```python
from build123d import *

# Parameters (mm, degrees)
SKETCH1_R                = 1.5
BOSS_EXTRUDE1_DEPTH      = 5
BOSS_EXTRUDE3_START      = -5
SKETCH3_R                = 1.5
BOSS_EXTRUDE3_DEPTH      = 5
BOSS_EXTRUDE5_DEPTH      = 6
BOSS_EXTRUDE5_DEPTH_BACK = 5
BOSS_EXTRUDE5_START      = -3
SKETCH5_R                = 1.5
SKETCH6_W                = 10
SKETCH6_H                = 5.12
CUT_EXTRUDE1_DEPTH       = 10
FILLET1_R                = 5


with BuildPart() as part:
    # Sketch1 → Boss-Extrude1 (new body)
    with BuildSketch(Plane.XY):
        with BuildLine():
            Line((-35.37698341, 4), (-15.37698341, 4))
            ThreePointArc((-15.37698341, 4), (-11.37698341, 0), (-15.37698341, -4))
            Line((-15.37698341, -4), (-35.37698341, -4))
            ThreePointArc((-35.37698341, -4), (-39.37698341, 0), (-35.37698341, 4))
        make_face()
        with Locations((-35.37698341, 0)):
            Circle(SKETCH1_R, mode=Mode.SUBTRACT)
        with Locations((-15.37698341, 0)):
            Circle(SKETCH1_R, mode=Mode.SUBTRACT)
    extrude(amount=BOSS_EXTRUDE1_DEPTH)

    # Sketch3 → Boss-Extrude3 (add)
    with BuildSketch(Plane.XY.offset(5).offset(BOSS_EXTRUDE3_START)):
        with BuildLine():
            Line((-55.37698341, -4), (-35.37698341, -4))
            ThreePointArc((-35.37698341, -4), (-39.37698341, 0), (-35.37698341, 4))
            Line((-35.37698341, 4), (-55.37698341, 4))
            ThreePointArc((-55.37698341, 4), (-59.37698341, 0), (-55.37698341, -4))
        make_face()
        with Locations((-55.37698341, 0)):
            Circle(SKETCH3_R, mode=Mode.SUBTRACT)
    extrude(amount=BOSS_EXTRUDE3_DEPTH)

    # Sketch5 → Boss-Extrude5 (add, two sides: drawn at the far end of the back side and taken through both)
    with BuildSketch(Plane.XY.offset(5).offset(BOSS_EXTRUDE5_START - BOSS_EXTRUDE5_DEPTH_BACK)):
        with BuildLine():
            Line((-44.37698341, -4), (-44.37698341, 4))
            Line((-44.37698341, 4), (-55.37698341, 4))
            ThreePointArc((-55.37698341, 4), (-59.37698341, 0), (-55.37698341, -4))
            Line((-55.37698341, -4), (-44.37698341, -4))
        make_face()
        with Locations((-55.37698341, 0)):
            Circle(SKETCH5_R, mode=Mode.SUBTRACT)
    extrude(amount=BOSS_EXTRUDE5_DEPTH + BOSS_EXTRUDE5_DEPTH_BACK)

    # Sketch6 → Cut-Extrude1 (cut)
    with BuildSketch(Plane(origin=(0, 4, 0), x_dir=(1, 0, 0), z_dir=(0, 1, 0))):
        with Locations((-54.37698341, -2.5)):
            Rectangle(SKETCH6_W, SKETCH6_H)
    extrude(amount=-CUT_EXTRUDE1_DEPTH, mode=Mode.SUBTRACT)

    # Fillet1
    # the kernel refuses this fillet: 5 mm, written as the material it takes off along each edge
    with BuildSketch(Plane(origin=(-44.37698341, -15.456439237, -3), x_dir=(0, 0, 1), z_dir=(0, 1, 0))) as fillet1_piece_1:
        with BuildLine():
            CenterArc((5, -4.582575695), FILLET1_R, 113.578178478, 66.421821522)
            Line((0, -4.582575695), (-0.1, -4.582575695))
            Line((-0.1, -4.582575695), (-0.1, 0))
            Line((-0.1, 0), (0, 0.1))
            ThreePointArc((0, 0.1), (1.5, 0.1), (2.96, 0.091651514))
            Line((2.96, 0.091651514), (3, 0))
        make_face()
    extrude(amount=30.912878475, mode=Mode.SUBTRACT)
    with BuildSketch(Plane(origin=(-44.37698341, -15.456439237, 8), x_dir=(-1, 0, 0), z_dir=(0, 1, 0))) as fillet1_piece_2:
        with BuildLine():
            CenterArc((4.582575695, -5), FILLET1_R, 90, 66.421821522)
            Line((0, -3), (-0.091651514, -2.96))
            ThreePointArc((-0.091651514, -2.96), (-0.1, -1.5), (-0.1, 0))
            Line((-0.1, 0), (0, 0.1))
            Line((0, 0.1), (4.582575695, 0.1))
            Line((4.582575695, 0.1), (4.582575695, 0))
        make_face()
    extrude(amount=30.912878475, mode=Mode.SUBTRACT)


solid = part.part
```
Geometry check sheet. Reference: the model listing, model coordinates, mm. A direction names the side the tool comes from. Give positions to 0.01 mm unless a question says otherwise; leave off trailing zeros. Loops run counter-clockwise (first coordinate to the right, second up) from the corner with the lowest first, then second, coordinate; pieces in that order, holes last. Notation, with made-up numbers: M -18.5,-24 L -7.5,-24 A15 ccw -7.5,-11 Z; hole C 43,-24.75 d4. An arc over 180 degrees is marked long. Write item = value, one per line. Start each with the question number.
1. Section check B-B, the plane z = 0.5. Enter the section's corners in (x, y), plus the area to 3 significant figures.
2. Go/stop test with flat-tipped pins: P1, Ø1.5, axis at y = -2.5, z = 6, coming from the +X side; P2, Ø1.5, axis at y = 0, z = -0.5, coming from the +X side; P3, Ø2.5, axis at x = -35.38, y = 0, coming from the -Z side; P4, Ø3.5, axis at x = -15.38, y = 0, coming from the -Z side. Record where each tip stops, or that it passes through.
3. Section check A-A, the plane y = 0. Enter the section's corners in (x, z), plus the area to 3 significant figures.
4. Section check C-C, the plane x = -56. Enter the section's corners in (y, z).
5. Tool access check on faces 5 (the face through (-28, 0, 5)), 6 (the face through (-53, 0, 5.06)), 7 (the face through (-53, 0, 8)), 8 (the face through (-28, 0, 0)), 9 (the face through (-36, -4, 2)). Record the directions out of +Z, -Z, +X, -X, +Y, -Y that give a thin tool (end or side, any length) a straight path to the whole face; none if there is none.
6. Section check D-D, the plane y = -2.5. Enter the section's corners in (x, z).
7. Thickness scan on probe 1 along Z at (x, y) = (-53.5, -3.5); probe 2 along X at (y, z) = (0.5, 3); probe 3 along X at (y, z) = (1.25, 4.75). Record the ranges inside material, lowest first.
8. Draft check along X on faces 1 (the face through (-11.378, 0.088, 2.465)), 2 (the face through (-35, 4, 2)), 3 (the face through (-53.946, 0.451, 6.509)), 4 (the face through (-53.946, 0.451, -1.551)). Enter one of: +X half, -X half, draft (parallel to the pull), parting line (faces both ways), or undercut.
Values follow:
q1.outline = M -49.38,-4 L -15.38,-4 A4 ccw -15.38,4 L -49.38,4 Z; hole C -35.38,0 d3; hole C -15.38,0 d3
q1.area = 283 mm^2
q2.P1 = -44.49
q2.P2 = -11.38
q2.P3 = through
q2.P4 = 0
q3.outline = M -59.38,-3 L -56.88,-3 L -56.88,-0.06 L -59.38,-0.06 Z; M -59.38,5.06 L -56.88,5.06 L -56.88,8 L -59.38,8 Z; M -53.88,-3 L -48.96,-3 A5 ccw -44.38,0 L -36.88,0 L -36.88,5 L -44.38,5 A5 ccw -48.96,8 L -53.88,8 L -53.88,5.06 L -49.38,5.06 L -49.38,-0.06 L -53.88,-0.06 Z; M -33.88,0 L -16.88,0 L -16.88,5 L -33.88,5 Z; M -13.88,0 L -11.38,0 L -11.38,5 L -13.88,5 Z
q3.area = 223 mm^2
q4.outline = M -3.95,-3 L -1.36,-3 L -1.36,-0.06 L -3.95,-0.06 Z; M -3.95,5.06 L -1.36,5.06 L -1.36,8 L -3.95,8 Z; M 1.36,-3 L 3.95,-3 L 3.95,-0.06 L 1.36,-0.06 Z; M 1.36,5.06 L 3.95,5.06 L 3.95,8 L 1.36,8 Z
q5.face_5 = +Z, +X, +Y, -Y
q5.face_6 = -X, +Y, -Y
q5.face_7 = +Z, +X, -X, +Y, -Y
q5.face_8 = -Z, +X, +Y, -Y
q5.face_9 = +Z, -Z, +X, -X, -Y
q6.outline = M -58.5,-3 L -48.96,-3 A5 ccw -44.38,0 L -12.25,0 L -12.25,5 L -44.38,5 A5 ccw -48.96,8 L -58.5,8 L -58.5,5.06 L -49.38,5.06 L -49.38,-0.06 L -58.5,-0.06 Z
q7.probe_1 = -3 to -0.06, 5.06 to 8
q7.probe_2 = -49.38 to -36.79, -33.96 to -16.79, -13.96 to -11.41
q7.probe_3 = -49.38 to -36.21, -34.55 to -16.21, -14.55 to -11.58
q8.face_1 = +X half
q8.face_2 = draft
q8.face_3 = undercut
q8.face_4 = undercut
